from build123d import *

# Parameters (mm, degrees)
ESQUISSE1_R        = 1.75
BOSS_EXTRU_1_DEPTH = 1.5
ESQUISSE2_W        = 76.5
ESQUISSE2_H        = 88
BOSS_EXTRU_2_DEPTH = 25


with BuildPart() as part:
    # Esquisse1 → Boss.-Extru.1 (new body)
    with BuildSketch(Plane.XY):
        with BuildLine():
            Line((72, 0), (72, 4.25))
            ThreePointArc((72, 4.25), (73.75, 6), (75.5, 4.25))
            Line((75.5, 4.25), (75.5, 0))
            Line((75.5, 0), (78, 0))
            Line((78, 0), (78, 111))
            Line((78, 111), (0, 111))
            Line((0, 111), (0, 0))
            Line((0, 0), (72, 0))
        make_face()
        with Locations((5, 106)):
            Circle(ESQUISSE1_R, mode=Mode.SUBTRACT)
    extrude(amount=BOSS_EXTRU_1_DEPTH)

    # Esquisse2 → Boss.-Extru.2 (add)
    with BuildSketch(Plane.XY.offset(1.5)):
        with Locations((39.75, 51)):
            Rectangle(ESQUISSE2_W, ESQUISSE2_H)
        Polygon((1.5, 111), (0, 111), (0, 0), (1.5, 0), (1.5, 7), (1.5, 95), align=None)
    extrude(amount=BOSS_EXTRU_2_DEPTH)


solid = part.part
Model file for the job. Use its own axes, mm. A direction names the side the tool comes from. Give positions to 0.01 mm unless a question says otherwise; leave off trailing zeros. Order: outer loops, then holes, each group sorted by start corner. A loop starts at its lowest first (then second) coordinate and runs counter-clockwise, first axis right, second up. Notation, with made-up numbers: (87.5, 59.5) - (141.5, 59.5) arc R19 cw to (141.5, 69.5) - close; hole circle Ø7 at (73, -5.5). An arc over 180 degrees is marked (long way). Return JSON: item names as keys, results as strings.
1) Flat gauge pins, fed straight in: P1, Ø12.5, axis at x = 43, z = 13.5, coming from the -Y side; P2, Ø2, axis at y = 3, z = 9.5, coming from the +X side; P3, Ø8, axis at x = 11.5, z = 12.5, coming from the +Y side; P4, Ø3, axis at x = 5, y = 106, coming from the +Z side. Where does each tip first touch, or does it go through?
Geometry says:
{"P1": "y = 7", "P2": "x = 1.5", "P3": "y = 95", "P4": "through"}
2) Cut at C-C, the plane x = 44. Give the cut face in (y, z).
Geometry says:
{"outline": "(0, 0) - (111, 0) - (111, 1.5) - (95, 1.5) - (95, 26.5) - (7, 26.5) - (7, 1.5) - (0, 1.5) - close"}
3) Cut at B-B, the plane y = 106. Give the cut face in (x, z), plus the area to 3 significant figures.
Geometry says:
{"outline": "(0, 0) - (3.25, 0) - (3.25, 1.5) - (1.5, 1.5) - (1.5, 26.5) - (0, 26.5) - close; (6.75, 0) - (78, 0) - (78, 1.5) - (6.75, 1.5) - close", "area": "149 mm²"}
4) Cut at D-D, the plane z = 8.25. Give the cut face in (x, y), plus the area to 3 significant figures.
Geometry says:
{"outline": "(0, 0) - (1.5, 0) - (1.5, 7) - (78, 7) - (78, 95) - (1.5, 95) - (1.5, 111) - (0, 111) - close", "area": "6,900 mm²"}
5) Probe line 1 (Y direction, x = 5, z = 0.9); line 2 (X direction, y = 106, z = 0.4); line 3 (X direction, y = 4, z = 13). List the from-to ranges inside material, lowest first. Write a range as from..to.
Geometry says:
{"line 1": "0..104.25, 107.75..111", "line 2": "0..3.25, 6.75..78", "line 3": "0..1.5"}
6) 3-axis set-ups, long thin cutter, end or side, ignore diameter. For faces 4 (the flat face through (39, 103, 1.5)), 5 (the flat face through (39.2, 111, 0.4)), 6 (the flat face through (39, 4, 1.5)): which of +Z, -Z, +X, -X, +Y, -Y reach the whole face in a straight line?
Geometry says:
{"face 4": "+Z, +X, +Y", "face 5": "+Z, -Z, +X, -X, +Y", "face 6": "+Z, +X, -Y"}
7) Pull direction Y, two halves, no side cores. Call faces 1 (the flat face through (39, 95, 14)), 2 (the flat face through (1.5, 103, 14)), 3 (the cylindrical face through (4.62, 104.29, 0.74)): pulls with the +Y half, pulls with the -Y half, needs draft (parallel to the pull), parting line crosses it, or undercut.
Geometry says:
{"face 1": "pulls with the +Y half", "face 2": "needs draft", "face 3": "undercut"}
8) Cut at A-A, the plane x = 5. Give the cut face in (y, z), plus the area to 3 significant figures.
Geometry says:
{"outline": "(0, 0) - (104.25, 0) - (104.25, 1.5) - (95, 1.5) - (95, 26.5) - (7, 26.5) - (7, 1.5) - (0, 1.5) - close; (107.75, 0) - (111, 0) - (111, 1.5) - (107.75, 1.5) - close", "area": "2,360 mm²"}
